```python
from build123d import *

# Parameters (mm, degrees)
EXTRUDE_1_DEPTH     = 4
FILLET_1_R          = 30
FILLET_2_R          = 30
SKETCH_4_R          = 1.65
CUT_EXTRUDE_3_DEPTH = 4
FILLET_4_R          = 10
FILLET_5_R          = 3
SKETCH_7_W          = 16
SKETCH_7_H          = 4
EXTRUDE_3_DEPTH     = 4
CUT_EXTRUDE_5_DEPTH = 4
FILLET_7_R          = 1
SKETCH_9_R          = 15
CUT_EXTRUDE_6_DEPTH = 10
SKETCH_10_R         = 2
CUT_EXTRUDE_7_DEPTH = 10
CHAMFER_1_SIZE      = 3
SKETCH_11_R         = 1.2
CUT_EXTRUDE_8_DEPTH = 10
SKETCH_12_R         = 1.5
CUT_EXTRUDE_9_DEPTH = 10


with BuildPart() as part:
    # 草图1 → 凸台-拉伸1 (new body)
    with BuildSketch(Plane(origin=(0, 0, 0), x_dir=(1, 0, 0), z_dir=(0, 1, 0))):
        with BuildLine():
            Line((-85, 80), (-35, 80))
            Line((-35, 80), (-35, 70))
            Line((-35, 70), (0, 36))
            ThreePointArc((0, 36), (25.455844123, -25.455844123), (-36, 0))
            Line((-36, 0), (-85, 70))
            Line((-85, 70), (-85, 80))
        make_face()
    extrude(amount=EXTRUDE_1_DEPTH)

    # 圆角1
    fillet_1_edges = [part.edges().sort_by_distance(p)[0] for p in [
        (0, 2, -36),
    ]]
    fillet(fillet_1_edges, radius=FILLET_1_R)

    # 圆角2
    fillet_2_edges = [part.edges().sort_by_distance(p)[0] for p in [
        (-36, 2, 0),
    ]]
    fillet(fillet_2_edges, radius=FILLET_2_R)

    # 草图4 → 切除-拉伸3 (cut)
    with BuildSketch(Plane(origin=(0, 4, 0), x_dir=(1, 0, 0), z_dir=(0, 1, 0))):
        with Locations(Location((-46, 76, 0), (0, 0, 270))):
            Circle(SKETCH_4_R)
        with Locations(Location((-74, 76, 0), (0, 0, 90))):
            Circle(SKETCH_4_R)
    extrude(amount=-CUT_EXTRUDE_3_DEPTH, mode=Mode.SUBTRACT)

    # 圆角4
    fillet_4_edges = [part.edges().sort_by_distance(p)[0] for p in [
        (-35, 2, -70),
        (-85, 2, -70),
    ]]
    fillet(fillet_4_edges, radius=FILLET_4_R)

    # 圆角5
    fillet_5_edges = [part.edges().sort_by_distance(p)[0] for p in [
        (-85, 2, -80),
        (-35, 2, -80),
    ]]
    fillet(fillet_5_edges, radius=FILLET_5_R)

    # 草图7 → 凸台-拉伸3 (add)
    with BuildSketch(Plane(origin=(0, 4, 0), x_dir=(1, 0, 0), z_dir=(0, 1, 0))):
        with Locations((-60, 82)):
            Rectangle(SKETCH_7_W, SKETCH_7_H)
    extrude(amount=-EXTRUDE_3_DEPTH)

    # 草图8 → 切除-拉伸5 (cut)
    with BuildSketch(Plane(origin=(0, 4, 0), x_dir=(1, 0, 0), z_dir=(0, 1, 0))):
        with BuildLine():
            Line((-50, 80), (-52, 80))
            ThreePointArc((-52, 80), (-51, 79), (-50, 80))
        make_face()
        with BuildLine():
            Line((-70, 80), (-68, 80))
            ThreePointArc((-68, 80), (-69, 79), (-70, 80))
        make_face()
    extrude(amount=-CUT_EXTRUDE_5_DEPTH, mode=Mode.SUBTRACT)

    # 圆角7
    fillet_7_edges = [part.edges().sort_by_distance(p)[0] for p in [
        (-52, 2, -84),
        (-68, 2, -84),
    ]]
    fillet(fillet_7_edges, radius=FILLET_7_R)

    # 草图9 → 切除-拉伸6 (cut)
    with BuildSketch(Plane(origin=(0, 4, 0), x_dir=(1, 0, 0), z_dir=(0, 1, 0))):
        with Locations(Location((0, 0, 0), (0, 0, 270))):
            Circle(SKETCH_9_R)
    extrude(amount=-CUT_EXTRUDE_6_DEPTH, mode=Mode.SUBTRACT)

    # 草图10 → 切除-拉伸7 (cut)
    with BuildSketch(Plane.XZ):
        with Locations(Location((29, 0, 0), (0, 0, 270))):
            Circle(SKETCH_10_R)
        with Locations(Location((-14.5, -25.11473671, 0), (0, 0, 270))):
            Circle(SKETCH_10_R)
        with Locations(Location((-14.5, 25.11473671, 0), (0, 0, 270))):
            Circle(SKETCH_10_R)
    extrude(amount=-CUT_EXTRUDE_7_DEPTH, mode=Mode.SUBTRACT)

    # 倒角1
    chamfer_1_edges = [part.edges().sort_by_distance(p)[0] for p in [
        (29, 4, 2),
        (-14.5, 4, -23.11473671),
        (-14.5, 4, 27.11473671),
    ]]
    chamfer(chamfer_1_edges, length=CHAMFER_1_SIZE)

    # 草图11 → 切除-拉伸8 (cut)
    with BuildSketch(Plane(origin=(0, 4, 0), x_dir=(1, 0, 0), z_dir=(0, 1, 0))):
        with Locations(Location((-29.401166302, 40.007142113, 0), (0, 0, 270))):
            Circle(SKETCH_11_R)
        with Locations(Location((-43.686880588, 54.004226358, 0), (0, 0, 270))):
            Circle(SKETCH_11_R)
    extrude(amount=-CUT_EXTRUDE_8_DEPTH, mode=Mode.SUBTRACT)

    # 草图12 → 切除-拉伸9 (cut)
    with BuildSketch(Plane(origin=(0, 4, 0), x_dir=(1, 0, 0), z_dir=(0, 1, 0))):
        with Locations(Location((-43.686880588, 54.004226358, 0), (0, 0, 270))):
            Circle(SKETCH_12_R)
        with Locations(Location((-29.401166302, 40.007142113, 0), (0, 0, 270))):
            Circle(SKETCH_12_R)
    extrude(amount=-CUT_EXTRUDE_9_DEPTH, mode=Mode.SUBTRACT)


solid = part.part
```
Could you check a few things on this model? Use its own coordinates, in mm. A direction names the side the tool comes from. Round coordinates to 2 decimals unless told otherwise and drop trailing zeros. Write each loop counter-clockwise with the first axis right and the second up, starting at its lowest first coordinate (ties: lowest second). Pieces come first, ordered by that corner, then holes. Notation, with made-up numbers: M -10.75,50.25 L -0.75,50.25 A14 ccw -0.75,73.25 Z; hole C 58,15 d5. An arc over 180 degrees is marked long. Write each question's results on one line, items separated by ' | '. Start each with the question number.
1. I'm going to push flat-ended pins straight in: pin 1 Ø6.5 at (x, z) = (-14.5, -25.11) entering from +Y; pin 2 Ø1.5 at (x, y) = (-49, 3.5) entering from -Z; pin 3 Ø1.5 at (y, z) = (3, 1.5) entering from -X. Where does each tip first touch, or does it pass through?
2. Imagine slicing it at D-D on z = -44.5. List the corners of the cut face in (x, y) for me.
3. On a 3-axis mill with a long thin cutter (end or side, diameter ignored), from which of +Z, -Z, +X, -X, +Y, -Y can I reach the whole of each face in a straight line? I mean faces 1 (the face through (-60, 2, -84)), 2 (the face through (-76, 2, -80)), 3 (the face through (-44, 2, -80)). Say none if no direction works.
4. Imagine slicing it at C-C on x = 0. List the corners of the cut face in (y, z) for me, and give its area (3 significant figures).
5. Imagine slicing it at B-B on y = 1.9. Count the separate pieces of the cut face and the enclosed holes in it, and give its area (3 significant figures).
6. Thinking about a two-plate mould opening in Z: for faces 4 (the face through (25.65, 1.97, 25.26)), 5 (the face through (27.048, 0.493, 0.434)), 6 (the face through (-35, 2, -76)), which applies, +Z half, -Z half, draft (parallel to the pull), parting line (faces both ways), or undercut?
7. Imagine slicing it at A-A on z = 13. List the corners of the cut face in (x, y) for me, and give its area (3 significant figures).
8. I need wall thicknesses on L1, parallel to X at y = 1.2, z = 0; L2, parallel to X at y = 0.3, z = 0; L3, parallel to Z at x = -74, y = 2.7. Which ranges of each line are inside material? Lowest first, please. Write a range as from..to.
Result sheet:
1) pin 1: stops at y = 2.25 | pin 2: stops at z = -80 | pin 3: stops at x = -36.83
2) outline: M -67.15,0 L -8.75,0 L -8.75,4 L -67.15,4 Z
3) face 1: -Z, +X, -X, +Y, -Y | face 2: -Z, -X, +Y, -Y | face 3: -Z, +X, +Y, -Y
4) outline: M 0,-37.86 L 4,-37.86 L 4,-15 L 0,-15 Z; M 0,15 L 4,15 L 4,36 L 0,36 Z | area: 175 mm^2
5) separate pieces: 1 | enclosed holes: 8 | area: 6,450 mm^2
6) face 4: parting line | face 5: undercut | face 6: draft
7) outline: M -33.57,0 L -7.48,0 L -7.48,4 L -33.57,4 Z; M 7.48,0 L 33.57,0 L 33.57,4 L 7.48,4 Z | area: 209 mm^2
8) L1: x = -37.1..-15, 15..26.8, 31.2..36 | L2: x = -37.1..-15, 15..27, 31..36 | L3: z = -80..-77.65, -74.35..-54.29
